```python
from build123d import *

# Parameters (mm, degrees)
SKETCH1_W           = 400
SKETCH1_H           = 120
BOSS_EXTRUDE1_DEPTH = 3
CUT_EXTRUDE1_REACH  = 210.828
CUT_EXTRUDE2_REACH  = 210.828
SKETCH3_R           = 2.5


with BuildPart() as part:
    # Sketch1 → Boss-Extrude1 (new body)
    with BuildSketch(Plane.XY):
        Rectangle(SKETCH1_W, SKETCH1_H)
    extrude(amount=BOSS_EXTRUDE1_DEPTH)

    # Sketch2 → Cut-Extrude1 (cut, up to next)
    with BuildSketch(Plane(origin=(0, 0, 0), x_dir=(-1, 0, 0), z_dir=(0, 0, -1)), mode=Mode.PRIVATE) as cut_extrude1_sk1:
        with BuildLine():
            Line((200, 60), (147.100505063, 60))
            ThreePointArc((147.100505063, 60), (149.77928909, 59.467156728), (152.050252532, 57.949747468))
            Line((152.050252532, 57.949747468), (188.050252532, 21.949747468))
            ThreePointArc((188.050252532, 21.949747468), (190.321215973, 20.432338209), (193, 19.899494937))
            Line((193, 19.899494937), (200, 19.899494937))
            Line((200, 19.899494937), (200, 60))
        make_face()
    cut_extrude1_tool1 = extrude(cut_extrude1_sk1.sketch, amount=-CUT_EXTRUDE1_REACH, mode=Mode.PRIVATE) & part.part
    # Sketch2 → Cut-Extrude1 (cut, up to next)
    with BuildSketch(Plane(origin=(0, 0, 0), x_dir=(-1, 0, 0), z_dir=(0, 0, -1)), mode=Mode.PRIVATE) as cut_extrude1_sk2:
        with BuildLine():
            Line((-152.050252532, 57.949747468), (-188.050252532, 21.949747468))
            ThreePointArc((-188.050252532, 21.949747468), (-190.321215973, 20.432338209), (-193, 19.899494937))
            Line((-193, 19.899494937), (-200, 19.899494937))
            Line((-200, 19.899494937), (-200, 60))
            Line((-200, 60), (-147.100505063, 60))
            ThreePointArc((-147.100505063, 60), (-149.77928909, 59.467156728), (-152.050252532, 57.949747468))
        make_face()
    cut_extrude1_tool2 = extrude(cut_extrude1_sk2.sketch, amount=-CUT_EXTRUDE1_REACH, mode=Mode.PRIVATE) & part.part
    add(cut_extrude1_tool1.solids().sort_by_distance((-182.75247, 44.458509, 0))[0], mode=Mode.SUBTRACT)
    add(cut_extrude1_tool2.solids().sort_by_distance((182.75247, 44.458509, 0))[0], mode=Mode.SUBTRACT)

    # Sketch3 → Cut-Extrude2 (cut, up to next)
    with BuildSketch(Plane.XY.offset(3), mode=Mode.PRIVATE) as cut_extrude2_sk1:
        with Locations((-80, 50)):
            Circle(SKETCH3_R)
    cut_extrude2_tool1 = extrude(cut_extrude2_sk1.sketch, amount=-CUT_EXTRUDE2_REACH, mode=Mode.PRIVATE) & part.part
    # Sketch3 → Cut-Extrude2 (cut, up to next)
    with BuildSketch(Plane.XY.offset(3), mode=Mode.PRIVATE) as cut_extrude2_sk2:
        with Locations((0, 50)):
            Circle(SKETCH3_R)
    cut_extrude2_tool2 = extrude(cut_extrude2_sk2.sketch, amount=-CUT_EXTRUDE2_REACH, mode=Mode.PRIVATE) & part.part
    # Sketch3 → Cut-Extrude2 (cut, up to next)
    with BuildSketch(Plane.XY.offset(3), mode=Mode.PRIVATE) as cut_extrude2_sk3:
        with Locations((0, -50)):
            Circle(SKETCH3_R)
    cut_extrude2_tool3 = extrude(cut_extrude2_sk3.sketch, amount=-CUT_EXTRUDE2_REACH, mode=Mode.PRIVATE) & part.part
    # Sketch3 → Cut-Extrude2 (cut, up to next)
    with BuildSketch(Plane.XY.offset(3), mode=Mode.PRIVATE) as cut_extrude2_sk4:
        with Locations((-80, -50)):
            Circle(SKETCH3_R)
    cut_extrude2_tool4 = extrude(cut_extrude2_sk4.sketch, amount=-CUT_EXTRUDE2_REACH, mode=Mode.PRIVATE) & part.part
    # Sketch3 → Cut-Extrude2 (cut, up to next)
    with BuildSketch(Plane.XY.offset(3), mode=Mode.PRIVATE) as cut_extrude2_sk5:
        with Locations((80, -50)):
            Circle(SKETCH3_R)
    cut_extrude2_tool5 = extrude(cut_extrude2_sk5.sketch, amount=-CUT_EXTRUDE2_REACH, mode=Mode.PRIVATE) & part.part
    # Sketch3 → Cut-Extrude2 (cut, up to next)
    with BuildSketch(Plane.XY.offset(3), mode=Mode.PRIVATE) as cut_extrude2_sk6:
        with Locations((80, 50)):
            Circle(SKETCH3_R)
    cut_extrude2_tool6 = extrude(cut_extrude2_sk6.sketch, amount=-CUT_EXTRUDE2_REACH, mode=Mode.PRIVATE) & part.part
    add(cut_extrude2_tool1.solids().sort_by_distance((-80, 50, 3))[0], mode=Mode.SUBTRACT)
    add(cut_extrude2_tool2.solids().sort_by_distance((0, 50, 3))[0], mode=Mode.SUBTRACT)
    add(cut_extrude2_tool3.solids().sort_by_distance((0, -50, 3))[0], mode=Mode.SUBTRACT)
    add(cut_extrude2_tool4.solids().sort_by_distance((-80, -50, 3))[0], mode=Mode.SUBTRACT)
    add(cut_extrude2_tool5.solids().sort_by_distance((80, -50, 3))[0], mode=Mode.SUBTRACT)
    add(cut_extrude2_tool6.solids().sort_by_distance((80, 50, 3))[0], mode=Mode.SUBTRACT)


solid = part.part
```
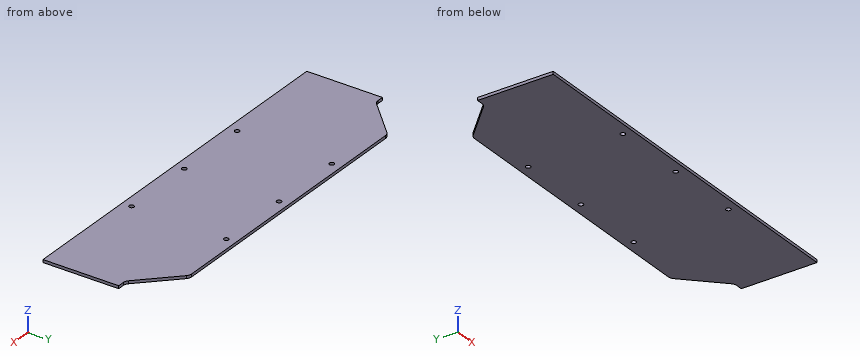
Check sheet for the modelled part. Datum: model origin and axes. Units: mm. Give positions to 0.01 mm unless a question says otherwise; leave off trailing zeros. Loops run counter-clockwise (first coordinate to the right, second up) from the corner with the lowest first, then second, coordinate; pieces in that order, holes last. Notation, with made-up numbers: (71, -30) - (78, -30) arc R19 cw to (78, 4) - close; hole circle Ø5 at (67, -0.75). An arc over 180 degrees is marked (long way). One line per question, with ' | ' between items. Start each with the question number.
1. Cross-section at A-A, the plane z = 2.1. Enter the section's corners in (x, y).
2. Gauge pin test, flat ends, axial feed: pin 1 Ø4 at (x, y) = (0, 50) entering from -Z; pin 2 Ø0.9 at (x, z) = (195.5, 2) entering from +Y. Record the tip position at first contact, or that the pin passes through.
3. Material ranges on line 1 along Y through (x, z) = (80, 1.6); line 2 along Y through (x, z) = (172, 0.4); line 3 along Y through (x, z) = (-161, 2), recorded low to high. Write a range as [from, to].
Check result:
1) outline: (-200, -60) - (200, -60) - (200, 19.9) - (193, 19.9) arc R7 cw to (188.05, 21.95) - (152.05, 57.95) arc R7 ccw to (147.1, 60) - (-147.1, 60) arc R7 ccw to (-152.05, 57.95) - (-188.05, 21.95) arc R7 cw to (-193, 19.9) - (-200, 19.9) - close; hole circle Ø5 at (-80, -50); hole circle Ø5 at (-80, 50); hole circle Ø5 at (0, -50); hole circle Ø5 at (0, 50); hole circle Ø5 at (80, -50); hole circle Ø5 at (80, 50)
2) pin 1: passes through | pin 2: stops at y = 19.9
3) line 1: y = [-60, -52.5], [-47.5, 47.5], [52.5, 60] | line 2: y = [-60, 38] | line 3: y = [-60, 49]
